```python
from build123d import *

# Parameters (mm, degrees)
CROQUIS1_W              = 216.14
CROQUIS1_H              = 126.8
SALIENTE_EXTRUIR1_DEPTH = 15.9
CROQUIS5_W              = 210.14
CROQUIS5_H              = 120.8
CORTAR_EXTRUIR2_DEPTH   = 7
CROQUIS3_R              = 46
CORTAR_EXTRUIR1_DEPTH   = 252.092711165
CROQUIS6_R              = 1.825
CROQUIS6_R_2            = 1.65
CORTAR_EXTRUIR3_DEPTH   = 252.092711165
SALIENTE_EXTRUIR2_DEPTH = 27.4
CORTAR_EXTRUIR4_DEPTH   = 253.082327028
CORTAR_EXTRUIR5_DEPTH   = 10
SALIENTE_EXTRUIR3_REACH = 254.082
SALIENTE_EXTRUIR4_DEPTH = 25
CROQUIS13_W             = 61.875090743
CROQUIS13_H             = 28
CORTAR_EXTRUIR7_DEPTH   = 7
CROQUIS16_W             = 12
CROQUIS16_H             = 9
CROQUIS16_W_2           = 16
CROQUIS16_H_2           = 13
CORTAR_EXTRUIR8_DEPTH   = 7.7
CHAFL_N1_SIZE           = 10
CROQUIS21_W             = 102
CROQUIS21_H             = 46
CORTAR_EXTRUIR10_DEPTH  = 253.608539048
CORTAR_EXTRUIR11_REACH  = 268.038
CROQUIS23_W             = 27.206677637
CROQUIS23_H             = 8.999999982
CORTAR_EXTRUIR12_DEPTH  = 253.607680361
CROQUIS25_W             = 24.206677637
CROQUIS25_H             = 4.236354688
CORTAR_EXTRUIR16_DEPTH  = 50
CROQUIS26_W             = 24.206677637
CROQUIS26_H             = 4.25
CORTAR_EXTRUIR17_DEPTH  = 50
CROQUIS31_W             = 20.435797251
CROQUIS31_H             = 32.708240737
CORTAR_EXTRUIR19_DEPTH  = 4.25
CORTAR_EXTRUIR20_REACH  = 255.179
CROQUIS32_W             = 39.355076343
CROQUIS32_H             = 27.206677637


with BuildPart() as part:
    # Croquis1 → Saliente-Extruir1 (new body)
    with BuildSketch(Plane(origin=(0, 0, 0), x_dir=(1, 0, 0), z_dir=(0, 1, 0))):
        with Locations((108.07, 63.4)):
            Rectangle(CROQUIS1_W, CROQUIS1_H)
    extrude(amount=SALIENTE_EXTRUIR1_DEPTH)

    # Croquis5 → Cortar-Extruir2 (cut)
    with BuildSketch(Plane(origin=(0, 15.9, 0), x_dir=(1, 0, 0), z_dir=(0, 1, 0))):
        with Locations((108.07, 63.4)):
            Rectangle(CROQUIS5_W, CROQUIS5_H)
    extrude(amount=-CORTAR_EXTRUIR2_DEPTH, mode=Mode.SUBTRACT)

    # Croquis3 → Cortar-Extruir1 (cut, through all)
    with BuildSketch(Plane(origin=(0, 15.9, 0), x_dir=(1, 0, 0), z_dir=(0, 1, 0))):
        with Locations((108.07, 15.808005153)):
            Circle(CROQUIS3_R)
    extrude(amount=-CORTAR_EXTRUIR1_DEPTH, mode=Mode.SUBTRACT)

    # Croquis6 → Cortar-Extruir3 (cut, through all)
    with BuildSketch(Plane(origin=(0, 0, 0), x_dir=(-1, 0, 0), z_dir=(0, -1, 0))):
        with Locations(Location((-196.658016439, 30.303322363, 0), (0, 0, 90))):
            Circle(CROQUIS6_R)
        with Locations(Location((-185.122851299, 63.713322363, 0), (0, 0, 90))):
            Circle(CROQUIS6_R)
        with Locations(Location((-31.017148701, 63.713322363, 0), (0, 0, 270))):
            Circle(CROQUIS6_R)
        with Locations(Location((-19.481983561, 30.303322363, 0), (0, 0, 270))):
            Circle(CROQUIS6_R)
        with Locations(Location((-53.066508219, 94.858322363, 0), (0, 0, 90))):
            Circle(CROQUIS6_R_2)
        with Locations(Location((-163.073491781, 94.858322363, 0), (0, 0, 270))):
            Circle(CROQUIS6_R_2)
    extrude(amount=-CORTAR_EXTRUIR3_DEPTH, mode=Mode.SUBTRACT)

    # Croquis7 → Saliente-Extruir2 (add)
    with BuildSketch(Plane.XZ):
        Polygon((216.14, 0), (213.14, 0), (213.14, -123.8), (3, -123.8), (3, 0), (0, 0), (0, -126.8), (216.14, -126.8), align=None)
    extrude(amount=SALIENTE_EXTRUIR2_DEPTH)

    # Croquis8 → Cortar-Extruir4 (cut, through all)
    with BuildSketch(Plane(origin=(216.14, 0, 0), x_dir=(0, 0, -1), z_dir=(1, 0, 0))):
        with BuildLine():
            Line((124.134269168, -27.4), (63.4, -27.4))
            ThreePointArc((63.4, -27.4), (93.767134584, -11.538522587), (124.134269168, -27.4))
        make_face()
    extrude(amount=-CORTAR_EXTRUIR4_DEPTH, mode=Mode.SUBTRACT)

    # Croquis9 → Cortar-Extruir5 (cut)
    with BuildSketch(Plane(origin=(0, 0, -126.8), x_dir=(-1, 0, 0), z_dir=(0, 0, -1))):
        Polygon((-216.14, -20.764005722), (-166.027655823, -27.4), (-216.14, -27.4), align=None)
        Polygon((-50.112344177, -27.4), (0, -27.4), (0, -20.764005722), align=None)
    extrude(amount=-CORTAR_EXTRUIR5_DEPTH, mode=Mode.SUBTRACT)

    # Saliente-Extruir3: up to this face of the body (flat: up to its plane)
    saliente_extruir3_end = Plane(part.part.faces().sort_by_distance((108.07, -12.927901237, -123.8))[0])
    # Croquis10 → Saliente-Extruir3 (add, up to the picked face)
    with BuildSketch(Plane(origin=(0, 0, -126.8), x_dir=(-1, 0, 0), z_dir=(0, 0, -1)), mode=Mode.PRIVATE) as saliente_extruir3_sk1:
        Polygon((-166.027655823, -27.4), (-132.196508219, -31.88), (-83.946508219, -31.88), (-50.112344177, -27.4), align=None)
    saliente_extruir3_tool1 = split(extrude(saliente_extruir3_sk1.sketch, amount=-SALIENTE_EXTRUIR3_REACH, mode=Mode.PRIVATE), bisect_by=saliente_extruir3_end, keep=Keep.BOTH, mode=Mode.PRIVATE)
    add(saliente_extruir3_tool1.solids().sort_by(Axis((108.070651, -29.332241, -126.8), (0, 0, 1)))[0])

    # Croquis11 → Saliente-Extruir4 (add)
    with BuildSketch(Plane.XY):
        Polygon((151.268460309, 15.9), (151.268460309, 0), (213.14, 0), (213.14, -27.4), (216.14, -27.4), (216.14, 15.9), align=None)
        Polygon((0.003551053, -27.4), (0.003551053, 15.9), (64.875090743, 15.9), (64.875090743, 0), (3.003551053, 0), (3.003551053, -27.4), align=None)
    extrude(amount=SALIENTE_EXTRUIR4_DEPTH)

    # Croquis13 → Cortar-Extruir7 (cut)
    with BuildSketch(Plane(origin=(0, 15.9, 0), x_dir=(1, 0, 0), z_dir=(0, 1, 0))):
        with Locations((33.937545372, -11)):
            Rectangle(CROQUIS13_W, CROQUIS13_H)
        with Locations((182.202454628, -11)):
            Rectangle(CROQUIS13_W, CROQUIS13_H)
    extrude(amount=-CORTAR_EXTRUIR7_DEPTH, mode=Mode.SUBTRACT)

    # Croquis16 → Cortar-Extruir8 (cut)
    with BuildSketch(Plane.XZ):
        with Locations((31.02016514, -63.713322363)):
            Rectangle(CROQUIS16_W, CROQUIS16_H)
        with Locations((19.485, -30.303322363)):
            Rectangle(CROQUIS16_W_2, CROQUIS16_H_2)
        Polygon((186.575628008, -82.591759265), (186.575966494, -99.591759262), (156.5759665, -99.592356589), (156.575777943, -90.122356591), (167.575777941, -90.122137571), (167.575628012, -82.592137572), align=None)
        Polygon((191.121505569, -59.211668748), (191.121684768, -68.211668746), (179.12168477, -68.211907677), (179.121505572, -59.211907679), align=None)
        Polygon((204.656224503, -36.801399255), (188.656224506, -36.801717829), (188.655965664, -23.801717832), (204.655965661, -23.801399257), align=None)
        Polygon((29.566508219, -99.593322363), (59.566508219, -99.593322363), (59.566508219, -90.123322363), (48.566508219, -90.123322363), (48.566508219, -82.593322363), (29.566508219, -82.593322363), align=None)
    extrude(amount=-CORTAR_EXTRUIR8_DEPTH, mode=Mode.SUBTRACT)

    # Chaflán1
    chafl_n1_edges = [part.edges().sort_by_distance(p)[0] for p in [
        (3, 12.4, -123.8),
        (213.14, 12.4, -123.8),
    ]]
    chamfer(chafl_n1_edges, length=CHAFL_N1_SIZE)

    # Croquis21 → Cortar-Extruir10 (cut, through all)
    with BuildSketch(Plane.XZ):
        with Locations((108.071569823, -53.123322363)):
            Rectangle(CROQUIS21_W, CROQUIS21_H)
    extrude(amount=-CORTAR_EXTRUIR10_DEPTH, mode=Mode.SUBTRACT)

    # Cortar-Extruir11: up to this face of the body (flat: up to its plane)
    cortar_extruir11_end = Plane(part.part.faces().sort_by_distance((44.566508219, 3.85, -99.593322363))[0])
    # Croquis22 → Cortar-Extruir11 (cut, up to the picked face)
    with BuildSketch(Plane(origin=(0, 0, -126.8), x_dir=(-1, 0, 0), z_dir=(0, 0, -1)), mode=Mode.PRIVATE) as cortar_extruir11_sk1:
        with BuildLine():
            Line((-177.076508219, 4.25), (-216.14, 4.25))
            Line((-216.14, 4.25), (-216.14, -4.75))
            Line((-216.14, -4.75), (-177.076508219, -4.75))
            ThreePointArc((-177.076508219, -4.75), (-172.576508219, -0.25), (-177.076508219, 4.25))
        make_face()
    cortar_extruir11_tool1 = split(extrude(cortar_extruir11_sk1.sketch, amount=-CORTAR_EXTRUIR11_REACH, mode=Mode.PRIVATE), bisect_by=cortar_extruir11_end, keep=Keep.BOTH, mode=Mode.PRIVATE)
    # Croquis22 → Cortar-Extruir11 (cut, up to the picked face)
    with BuildSketch(Plane(origin=(0, 0, -126.8), x_dir=(-1, 0, 0), z_dir=(0, 0, -1)), mode=Mode.PRIVATE) as cortar_extruir11_sk2:
        with BuildLine():
            Line((-0.001303888, -4.756822615), (-39.06479559, -4.754356466))
            ThreePointArc((-39.06479559, -4.754356466), (-43.564511488, -0.254072381), (-39.064227404, 4.245643517))
            Line((-39.064227404, 4.245643517), (-0.000735701, 4.243177367))
            Line((-0.000735701, 4.243177367), (-0.001303888, -4.756822615))
        make_face()
    cortar_extruir11_tool2 = split(extrude(cortar_extruir11_sk2.sketch, amount=-CORTAR_EXTRUIR11_REACH, mode=Mode.PRIVATE), bisect_by=cortar_extruir11_end, keep=Keep.BOTH, mode=Mode.PRIVATE)
    add(cortar_extruir11_tool1.solids().sort_by(Axis((194.829267, -0.25, -126.8), (0, 0, 1)))[0], mode=Mode.SUBTRACT)
    add(cortar_extruir11_tool2.solids().sort_by(Axis((21.311752, -0.255477, -126.8), (0, 0, 1)))[0], mode=Mode.SUBTRACT)

    # Croquis23 → Cortar-Extruir12 (cut, through all)
    with BuildSketch(Plane(origin=(0.001003581, 6.3e-08, 0), x_dir=(0, 0, -1), z_dir=(0.9999999980071865, 6.3131823435647e-05, 0))):
        with Locations((113.196661182, -0.263645312)):
            Rectangle(CROQUIS23_W, CROQUIS23_H)
    extrude(amount=-CORTAR_EXTRUIR12_DEPTH, mode=Mode.SUBTRACT)

    # Croquis25 → Cortar-Extruir16 (cut)
    with BuildSketch(Plane.ZY):
        with Locations((-111.696661182, 2.118177344)):
            Rectangle(CROQUIS25_W, CROQUIS25_H)
    extrude(amount=-CORTAR_EXTRUIR16_DEPTH, mode=Mode.SUBTRACT)

    # Croquis26 → Cortar-Extruir17 (cut)
    with BuildSketch(Plane(origin=(216.14, 0, 0), x_dir=(0, 0, -1), z_dir=(1, 0, 0))):
        with Locations((111.696661182, 2.125)):
            Rectangle(CROQUIS26_W, CROQUIS26_H)
    extrude(amount=-CORTAR_EXTRUIR17_DEPTH, mode=Mode.SUBTRACT)

    # Croquis31 → Cortar-Extruir19 (cut)
    with BuildSketch(Plane.XZ):
        with Locations((176.357898626, -107.445879632)):
            Rectangle(CROQUIS31_W, CROQUIS31_H)
    extrude(amount=-CORTAR_EXTRUIR19_DEPTH, mode=Mode.SUBTRACT)

    # Cortar-Extruir20: up to this face of the body (flat: up to its plane)
    cortar_extruir20_end = Plane(part.part.faces().sort_by_distance((44.676749051, 4.236354688, -111.696661182))[0])
    # Croquis32 → Cortar-Extruir20 (cut, up to the picked face)
    with BuildSketch(Plane(origin=(-0.00026788, 4.243177304, 0), x_dir=(0.9999999980071865, 6.313182343619669e-05, 0), z_dir=(6.313182343619669e-05, -0.9999999980071865, 0)), mode=Mode.PRIVATE) as cortar_extruir20_sk1:
        with Locations((19.676227302, -113.196661182)):
            Rectangle(CROQUIS32_W, CROQUIS32_H)
    cortar_extruir20_tool1 = split(extrude(cortar_extruir20_sk1.sketch, amount=CORTAR_EXTRUIR20_REACH, mode=Mode.PRIVATE), bisect_by=cortar_extruir20_end, keep=Keep.BOTH, mode=Mode.PRIVATE)
    add(cortar_extruir20_tool1.solids().sort_by(Axis((19.675959, 4.244419, -113.196661), (6.313182343619669e-05, -0.9999999980071865, 0)))[0], mode=Mode.SUBTRACT)


solid = part.part
```
Design review of the part built by this model. Coordinates are the model's own, in mm. A direction names the side the tool comes from. Coordinates: 2 decimals unless noted, no trailing zeros. Order: outer loops, then holes, each group sorted by start corner. A loop starts at its lowest first (then second) coordinate and runs counter-clockwise, first axis right, second up.
1) Wall thickness on line 1 along X through (y, z) = (4, -66); line 2 along X through (y, z) = (-2, -20); line 3 along Z through (x, y) = (56, 7.5): over which ranges is each line inside the solid? List them lowest first.
2) Take a section at B-B, the plane y = -23.5. State how many separate pieces and enclosed holes the cut face has, and give its area (3 significant figures).
3) Take a section at C-C, the plane x = 100. Give the boundary of the cut face in (y, z), and give its area (3 significant figures).
4) Clearance check with flat-ended pins moving along their axes: pin 1 (2 mm diameter, centred on y = 2.5, z = -116, fed in from -X); pin 2 (2 mm diameter, centred on x = 63, z = -79.5, fed in from -Y); pin 3 (0.9 mm diameter, centred on x = 2, z = -15, fed in from -Y). State where each tip first meets the part, or that it passes through.
5) Take a section at A-A, the plane z = 15.5. Give the boundary of the cut face in (x, y), and give its area (3 significant figures).
6) Mouldability with a two-part tool opening along X and no side actions: class faces 4 (the flat face through (166.14, 2, -112)), 5 (the cylindrical face through (62.074, 4.512, -15.233)), 6 (the flat face through (31, 7.7, -66)), 7 (the flat face through (0, -5, -48)) as +X half, -X half, draft (parallel to the pull), parting line (faces both ways), or undercut.
7) For faces 1 (the flat face through (107, 12, -123.8)), 2 (the flat face through (159.072, 4, -53)), 3 (the flat face through (19, 4, -23.803)), list the 3-axis set-ups (+Z, -Z, +X, -X, +Y, -Y) from which the entire face can be reached by the end or side of a thin tool; tool diameter is ignored.
Returned:
1. line 1: x = 0 to 25.02, 37.02 to 57.07, 159.07 to 179.12, 191.12 to 216.14
1. line 2: x = 0 to 3, 213.14 to 216.14
1. line 3: z = -126.8 to -99.59, -90.12 to 25
2. separate pieces: 3
2. enclosed holes: 0
2. area: 1,070 mm2
3. outline: (-31.88, -126.8) - (15.9, -126.8) - (15.9, -123.8) - (8.9, -123.8) - (8.9, -76.12) - (0, -76.12) - (0, -123.8) - (-26.93, -123.8) arc R37 cw to (-27.4, -124.13) - (-27.4, -123.8) - (-31.88, -123.8) - close
3. area: 568 mm2
4. pin 1: stops at x = 50
4. pin 2: stops at y = 0
4. pin 3: stops at y = -27.4
5. outline: (0, -27.4) - (3, -27.4) - (3, 0) - (64.88, 0) - (64.88, 8.9) - (3, 8.9) - (3, 15.9) - (0, 15.9) - close; (151.27, 0) - (213.14, 0) - (213.14, -27.4) - (216.14, -27.4) - (216.14, 15.9) - (213.14, 15.9) - (213.14, 8.9) - (151.27, 8.9) - close
5. area: 1,360 mm2
6. face 4: +X half
6. face 5: undercut
6. face 6: undercut
6. face 7: -X half
7. face 1: +Z, +Y
7. face 2: +Y, -Y
7. face 3: -Y
